from build123d import *

# Parameters (mm, degrees)
BOSS_EXTRUDE1_DEPTH = 5
SKETCH2_R           = 2.5
BOSS_EXTRUDE2_DEPTH = 17


with BuildPart() as part:
    # Sketch1 → Boss-Extrude1 (new, symmetric)
    with BuildSketch(Plane.XY):
        Polygon((0, -2.9), (0, 2.9), (-0.4, 2.9), (-0.4, 4.95), (-2.4, 4.95), (-4, 2.9), (-4, -2.9), (-2.4, -4.95), (-0.4, -4.95), (-0.4, -2.9), align=None)
    extrude(amount=BOSS_EXTRUDE1_DEPTH, both=True)

    # Sketch2 → Boss-Extrude2 (add)
    with BuildSketch(Plane(origin=(0, 0, 0), x_dir=(0, 0, -1), z_dir=(1, 0, 0))):
        Circle(SKETCH2_R)
    extrude(amount=BOSS_EXTRUDE2_DEPTH)


solid = part.part
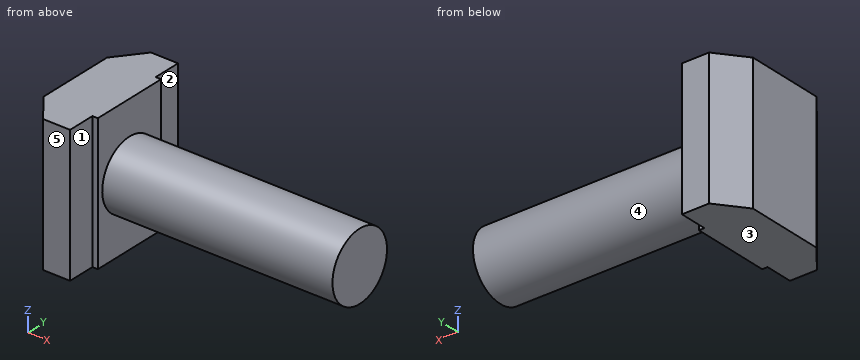
Input: part model. Units: mm. Frame: model coordinates. Face numbers are marked on the shaded views. A direction names the side the tool comes from. Coordinates: 2 decimals unless noted, no trailing zeros. Loops run counter-clockwise (first coordinate to the right, second up) from the corner with the lowest first, then second, coordinate; pieces in that order, holes last.
(1) First-contact query: pin 1 Ø1 at (y, z) = (4, -2.5) entering from -X; pin 2 Ø1 at (x, z) = (10, 2) entering from -Y; pin 3 Ø1 at (y, z) = (4, -0.5) entering from +X. Flat tips, straight axial feed; report the tip coordinate or a pass-through.
(2) Section C-C on z = 0. Return the cut outline in (x, y), then the cut area to 3 significant figures.
(3) Material intervals for probe 1 along X at (y, z) = (1.25, 4.25); probe 2 along Y at (x, z) = (2.25, -0.5), sorted ascending.
(4) Section D-D on x = 11.5. Return the cut outline in (y, z), then the cut area to 3 significant figures.
(5) Section B-B on y = 0. Return the cut outline in (x, z).
(6) Set-up query: the marked faces 1, 2, 3, 4 and 5. Return all of +Z, -Z, +X, -X, +Y, -Y with unobstructed straight access to the full face (end or side cutting, diameter ignored); none if empty.
(7) Section A-A on z = 3. Return the cut outline in (x, y), then the cut area to 3 significant figures.
Data:
1. pin 1: stops at x = -3.53
1. pin 2: stops at y = -2
1. pin 3: stops at x = -0.4
2. outline: (-4, -2.9) - (-2.4, -4.95) - (-0.4, -4.95) - (-0.4, -2.9) - (0, -2.9) - (0, -2.5) - (17, -2.5) - (17, 2.5) - (0, 2.5) - (0, 2.9) - (-0.4, 2.9) - (-0.4, 4.95) - (-2.4, 4.95) - (-4, 2.9) - close
2. area: 120 mm2
3. probe 1: x = -4 to 0
3. probe 2: y = -2.45 to 2.45
4. outline: circle Ø5 at (0, 0)
4. area: 19.6 mm2
5. outline: (-4, -5) - (0, -5) - (0, -2.5) - (17, -2.5) - (17, 2.5) - (0, 2.5) - (0, 5) - (-4, 5) - close
6. face 1: +Z, -Z, +X, -Y
6. face 2: +Z, -Z, +X, +Y
6. face 3: -Z, +X, -X, +Y, -Y
6. face 4: +X
6. face 5: +Z, -Z, +X, -X, -Y
7. outline: (-4, -2.9) - (-2.4, -4.95) - (-0.4, -4.95) - (-0.4, -2.9) - (0, -2.9) - (0, 2.9) - (-0.4, 2.9) - (-0.4, 4.95) - (-2.4, 4.95) - (-4, 2.9) - close
7. area: 34.7 mm2
